For this review, take the finished solid that the model builds, in its own axes (mm). A direction names the side the tool comes from. Coordinates: 2 decimals unless noted, no trailing zeros. Write each loop counter-clockwise with the first axis right and the second up, starting at its lowest first coordinate (ties: lowest second). Pieces come first, ordered by that corner, then holes. Notation, with made-up numbers: (45.5, 12) -> (59.5, 12) arc R27 ccw to (59.5, 37) -> close; hole circle Ø3 at (-33.5, 84.25). An arc over 180 degrees is marked (long way). Put each result on its own line as item: value. Start each with the question number.
Item 1: For faces 4 (the flat face through (25.4, 125, -38)), 5 (the flat face through (3.175, 125, -38)), list the 3-axis set-ups (+Z, -Z, +X, -X, +Y, -Y) from which the entire face can be reached by the end or side of a thin tool; tool diameter is ignored.
Item 2: Consider section C-C on y = 225.5. Give the boundary of the cut face in (x, z) (3 decimals).
Item 3: The part is to be moulded in two halves that separate along X. For faces 1 (the flat face through (22.225, 125, -38)), 2 (the flat face through (2, 254, -41)), 3 (the flat face through (0, 125, -39)), say which applies: +X half, -X half, draft (parallel to the pull), parting line (faces both ways), or undercut.
Item 4: Consider section B-B on x = 15. Give the boundary of the cut face in (y, z) (3 decimals), and give its area (3 significant figures).
Item 5: Consider section A-A on z = -39. Give the boundary of the cut face in (x, y) (3 decimals).
Item 6: Insertion check: P1, Ø10, axis at x = 19.5, y = 171.5, coming from the +Z side. The pin has a flat end and moves straight along its axis. Give the tip position at first contact, or say it passes through.
Item 7: To check wall thickness, follow L1, parallel to Z at x = 9.75, y = 132.5 (3 decimals); L2, parallel to X at y = 84, z = -57 (3 decimals). State the ranges of each line that lie inside material, in increasing order.
```python
from build123d import *

# Parameters (mm, degrees)
SKETCH1_W           = 3.175
SKETCH1_H           = 69.85
BOSS_EXTRUDE1_DEPTH = 254


with BuildPart() as part:
    # Sketch1 → Boss-Extrude1 (new body)
    with BuildSketch(Plane(origin=(0, 0, 0), x_dir=(1, 0, 0), z_dir=(0, 1, 0))):
        with Locations((1.5875, 38.1)):
            Rectangle(SKETCH1_W, SKETCH1_H)
        Polygon((3.175, 3.175), (0, 3.175), (0, 0), (25.4, 0), (25.4, 3.175), (22.225, 3.175), align=None)
        with Locations((23.8125, 38.1)):
            Rectangle(SKETCH1_W, SKETCH1_H)
        Polygon((25.4, 76.2), (0, 76.2), (0, 73.025), (3.175, 73.025), (22.225, 73.025), (25.4, 73.025), align=None)
    extrude(amount=BOSS_EXTRUDE1_DEPTH)


solid = part.part
```
Return value:
1. face 4: +Z, -Z, +X, +Y, -Y
1. face 5: +Y, -Y
2. outline: (0, -76.2) -> (25.4, -76.2) -> (25.4, 0) -> (0, 0) -> close; hole (3.175, -73.025) -> (22.225, -73.025) -> (22.225, -3.175) -> (3.175, -3.175) -> close
3. face 1: undercut
3. face 2: draft
3. face 3: -X half
4. outline: (0, -76.2) -> (254, -76.2) -> (254, -73.025) -> (0, -73.025) -> close; (0, -3.175) -> (254, -3.175) -> (254, 0) -> (0, 0) -> close
4. area: 1,610 mm^2
5. outline: (0, 0) -> (3.175, 0) -> (3.175, 254) -> (0, 254) -> close; (22.225, 0) -> (25.4, 0) -> (25.4, 254) -> (22.225, 254) -> close
6. P1: z = 0
7. L1: -76.2 to -73.025, -3.175 to 0
7. L2: 0 to 3.175, 22.225 to 25.4
